from build123d import *

# Parameters (mm, degrees)
CROQUIS1_R              = 16
SALIENTE_EXTRUIR1_DEPTH = 15
CROQUIS2_R              = 11
CORTAR_EXTRUIR1_DEPTH   = 10
CROQUIS3_R              = 5
CORTAR_EXTRUIR2_DEPTH   = 5
CHAFL_N1_SIZE           = 1
REDONDEO1_R             = 0.5


with BuildPart() as part:
    # Croquis1 → Saliente-Extruir1 (new body)
    with BuildSketch(Plane.XY):
        Circle(CROQUIS1_R)
    extrude(amount=SALIENTE_EXTRUIR1_DEPTH)

    # Croquis2 → Cortar-Extruir1 (cut)
    with BuildSketch(Plane.XY.offset(15)):
        Circle(CROQUIS2_R)
    extrude(amount=-CORTAR_EXTRUIR1_DEPTH, mode=Mode.SUBTRACT)

    # Croquis3 → Cortar-Extruir2 (cut)
    with BuildSketch(Plane.XY.offset(5)):
        Circle(CROQUIS3_R)
    extrude(amount=-CORTAR_EXTRUIR2_DEPTH, mode=Mode.SUBTRACT)

    # Chaflán1
    chafl_n1_edges = [part.edges().sort_by_distance(p)[0] for p in [
        (-11, 0, 15),
    ]]
    chamfer(chafl_n1_edges, length=CHAFL_N1_SIZE)

    # Redondeo1
    redondeo1_edges = [part.edges().sort_by_distance(p)[0] for p in [
        (-5, 0, 5),
        (-5, 0, 0),
        (-16, 0, 0),
        (-16, 0, 15),
        (-11, 0, 5),
    ]]
    fillet(redondeo1_edges, radius=REDONDEO1_R)


solid = part.part
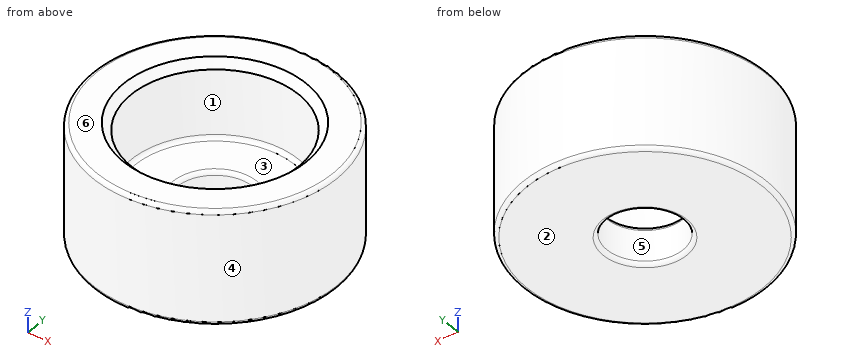
Check sheet for the modelled part. Datum: model origin and axes. Units: mm. Face numbers are marked on the shaded views. A direction names the side the tool comes from. Give positions to 0.01 mm unless a question says otherwise; leave off trailing zeros. Loops run counter-clockwise (first coordinate to the right, second up) from the corner with the lowest first, then second, coordinate; pieces in that order, holes last. Notation, with made-up numbers: M 50,-20 L 67,-20 A20 cw 67,19 Z; hole C 55,-30.75 d5. An arc over 180 degrees is marked long. Return JSON: item names as keys, results as strings. Group by question number.
1. Go/stop test with flat-tipped pins: pin 1 (8 mm diameter, centred on y = -9.5, z = 12.5, fed in from -X) (3 decimals); pin 2 (1.5 mm diameter, centred on x = 2.5, z = 8.5, fed in from -Y). Record where each tip stops, or that it passes through.
2. Cross-section at C-C on z = 8.25. Record the boundary of the cut face in (x, y).
3. Cross-section at A-A on x = 0. Record the boundary of the cut face in (y, z).
4. Thickness scan on L1, parallel to Y at x = 0, z = 10.25; L2, parallel to Y at x = 0, z = 3.75; L3, parallel to Z at x = 4, y = 5. Record the ranges inside material, lowest first.
5. Mould release check, pull along Y, two halves, no side actions. Record for the marked faces 3, 4, 5 and 6: released by +Y, released by -Y, zero draft, split by the parting line, or undercut.
6. Tool access check on the marked faces 1 and 2. Record the directions out of +Z, -Z, +X, -X, +Y, -Y that give a thin tool (end or side, any length) a straight path to the whole face; none if there is none.
Return value:
{
 "1": {"pin 1": "x = -15.025", "pin 2": "y = -15.9"},
 "2": {"outline": "C 0,0 d32; hole C 0,0 d22"},
 "3": {"outline": "M -16,0.5 A0.5 ccw -15.5,0 L -5.5,0 A0.5 ccw -5,0.5 L -5,4.5 A0.5 ccw -5.5,5 L -10.5,5 A0.5 cw -11,5.5 L -11,14 L -12,15 L -15.5,15 A0.5 ccw -16,14.5 Z; M 5,0.5 A0.5 ccw 5.5,0 L 15.5,0 A0.5 ccw 16,0.5 L 16,14.5 A0.5 ccw 15.5,15 L 12,15 L 11,14 L 11,5.5 A0.5 cw 10.5,5 L 5.5,5 A0.5 ccw 5,4.5 Z"},
 "4": {"L1": "-16 to -11, 11 to 16", "L2": "-16 to -5, 5 to 16", "L3": "0 to 5"},
 "5": {"face 3": "undercut", "face 4": "split by the parting line", "face 5": "undercut", "face 6": "zero draft"},
 "6": {"face 1": "+Z", "face 2": "-Z, +X, -X, +Y, -Y"}
}
